from build123d import *

# Parameters (mm, degrees)
SKETCH1_W           = 21.18343152
SKETCH1_H           = 2.7
BOSS_EXTRUDE1_DEPTH = 3


with BuildPart() as part:
    # Sketch1 → Boss-Extrude1 (new body)
    with BuildSketch(Plane(origin=(0, 0, 0), x_dir=(1, 0, 0), z_dir=(0, 1, 0))):
        Polygon((44.226000001, 0), (73.910000001, 0), (73.910000001, 3), (98.12973499, 3), (94.59216997, 16.202372389), (97.489947449, 16.978829524), (93.72803317, 31.018484749), (90.830255691, 30.242027613), (87.145987125, 43.99190509), (90.043764604, 44.768362225), (86.281850324, 58.808017449), (83.384072846, 58.031560314), (79.69980428, 71.781437791), (82.597581759, 72.557894926), (78.835667479, 86.59755015), (75.93789, 85.821093015), (72.253621435, 99.570970491), (75.151398913, 100.347427627), (71.389484634, 114.387082851), (68.491707155, 113.610625716), (64.150294558, 129.812998105), (64.150294558, 143.970140962), (67.150294558, 143.970140962), (67.150294558, 158.427283819), (64.150294558, 158.427283819), (64.150294558, 172.584426676), (67.150294558, 172.584426676), (67.150294558, 187.041569533), (64.150294558, 187.041569533), (64.150294558, 201.19871239), (67.150294558, 201.19871239), (67.150294558, 215.655855248), (64.150294558, 215.655855248), (64.150294558, 229.812998105), (-64.150294558, 229.812998105), (-64.150294558, 215.655855248), (-67.150294558, 215.655855248), (-67.150294558, 201.19871239), (-64.150294558, 201.19871239), (-64.150294558, 187.041569533), (-67.150294558, 187.041569533), (-67.150294558, 172.584426676), (-64.150294558, 172.584426676), (-64.150294558, 158.427283819), (-67.150294558, 158.427283819), (-67.150294558, 143.970140962), (-64.150294558, 143.970140962), (-64.150294558, 129.812998105), (-68.491707155, 113.610625716), (-71.389484634, 114.387082851), (-75.151398913, 100.347427627), (-72.253621435, 99.570970491), (-75.93789, 85.821093015), (-78.835667479, 86.59755015), (-82.597581759, 72.557894926), (-79.69980428, 71.781437791), (-83.384072846, 58.031560314), (-86.281850324, 58.808017449), (-90.043764604, 44.768362225), (-87.145987125, 43.99190509), (-90.830255691, 30.242027613), (-93.72803317, 31.018484749), (-97.489947449, 16.978829524), (-94.59216997, 16.202372389), (-98.12973499, 3), (-73.910000001, 3), (-73.910000001, 0), (-44.226000001, 0), (-44.226000001, 3), (-14.842, 3), (-14.842, 0), (14.842, 0), (14.842, 3), (44.226000001, 3), align=None)
        with Locations((-32.075147279, 149.812998105)):
            Rectangle(SKETCH1_W, SKETCH1_H, mode=Mode.SUBTRACT)
        with Locations((32.075147279, 149.812998105)):
            Rectangle(SKETCH1_W, SKETCH1_H, mode=Mode.SUBTRACT)
    extrude(amount=BOSS_EXTRUDE1_DEPTH)


solid = part.part
Source: CAD feature listing. Evaluate the final solid. Frame: model axes, mm. Give positions to 0.01 mm unless a question says otherwise; leave off trailing zeros. Write each loop counter-clockwise with the first axis right and the second up, starting at its lowest first coordinate (ties: lowest second). Pieces come first, ordered by that corner, then holes. Notation, with made-up numbers: (-24.5, 34) -> (31.5, 34) arc R19 cw to (31.5, 68) -> close; hole circle Ø9 at (1.25, 9). An arc over 180 degrees is marked (long way). Return JSON: item names as keys, results as strings. Group by question number.
1. Section D-D, the plane z = -64.5. Output: boundary loops of the cut face in (x, y), then the cut area to 3 significant figures.
2. Material intervals for line 1 (Z direction, x = 33.5, y = 0.4); line 2 (X direction, y = 2.15, z = -178.5); line 3 (X direction, y = 2.9, z = -170), sorted ascending. Write a range as from..to.
3. Section A-A, the plane x = 40. Output: boundary loops of the cut face in (y, z).
4. Pin query (flat end, axial travel): pin 1 Ø0.9 at (y, z) = (1, -205) entering from -X; pin 2 Ø0.9 at (x, y) = (82, 1) entering from +Z; pin 3 Ø0.9 at (y, z) = (2, -1) entering from +X. Return the tip coordinate at first contact, or that it passes through.
5. Section C-C, the plane z = -161.5. Output: boundary loops of the cut face in (x, y).
6. Section B-B, the plane y = 2.5. Count the separate pieces of the cut face and the enclosed holes in it, then the cut area to 3 significant figures.
Determined:
{
 "1": {"outline": "(-81.65, 0) -> (81.65, 0) -> (81.65, 3) -> (-81.65, 3) -> close", "area": "490 mm2"},
 "2": {"line 1": "z = -229.81..-151.16, -148.46..-3", "line 2": "x = -67.15..67.15", "line 3": "x = -64.15..64.15"},
 "3": {"outline": "(0, -229.81) -> (3, -229.81) -> (3, -151.16) -> (0, -151.16) -> close; (0, -148.46) -> (3, -148.46) -> (3, -3) -> (0, -3) -> close"},
 "4": {"pin 1": "stops at x = -67.15", "pin 2": "stops at z = -3", "pin 3": "stops at x = 73.91"},
 "5": {"outline": "(-64.15, 0) -> (64.15, 0) -> (64.15, 3) -> (-64.15, 3) -> close"},
 "6": {"separate pieces": "1", "enclosed holes": "2", "area": "34,200 mm2"}
}
